Input: part model. Units: mm. Frame: model coordinates. A direction names the side the tool comes from. Round coordinates to 2 decimals unless told otherwise and drop trailing zeros. Order: outer loops, then holes, each group sorted by start corner. A loop starts at its lowest first (then second) coordinate and runs counter-clockwise, first axis right, second up.
Item 1: Cut plane B-B on x = 0. Output: boundary loops of the cut face in (y, z) (3 decimals).
Item 2: First-contact query: pin 1 (6 mm diameter, centred on x = 23.5, y = 11, fed in from +Z); pin 2 (10 mm diameter, centred on y = -2, z = -2, fed in from +X); pin 3 (4 mm diameter, centred on x = -15.5, z = 14, fed in from -Y). Flat tips, straight axial feed; report the tip coordinate or a pass-through.
Item 3: Cut plane A-A on x = 40.5. Output: boundary loops of the cut face in (y, z).
Item 4: Line query: L1, parallel to Y at x = 40, z = -12; L2, parallel to Y at x = 6.5, z = 0; L3, parallel to Y at x = 31, z = 0. Output: solid intervals per line, ascending.
Item 5: Reachability of faces 1 (the conical face through (41.73, 26.92, -0.07)), 2 (the cylindrical face through (42.64, -20.24, 12.9)), 3 (the cylindrical face through (20.012, -11.49, -10.156)) from +Z, -Z, +X, -X, +Y, -Y: full face, straight path, thin tool, end or side. Return the list, or none.
Item 6: Mould query, pull axis Z, two halves, no side actions, for faces 4 (the flat face through (47, -10, -3)), 5 (the cylindrical face through (6.78, 14.36, 34.64)), 6 (the flat face through (-21.5, 24, 8)), 7 (the flat face through (38, -11, 10)). Classes: released by +Z, released by -Z, zero draft, split by the parting line, or undercut.
```python
from build123d import *

# Parameters (mm, degrees)
SKETCH4_R          = 13.125
CUT_EXTRUDE1_DEPTH = 45
FILLET1_R          = 0.4


with BuildPart() as part:
    # Sketch1 → Base-Revolve (revolve)
    with BuildSketch(Plane.XY, mode=Mode.PRIVATE) as base_revolve_sk:
        Polygon((-23, 0), (-23, 37.5), (35.741669751, 37.5), (47, 31), (47, 24), (38, 24), (38, 14), (47, 14), (47, 10), (34, 10), (34, 6), (25, 6), (21.535898385, 0), align=None)
    revolve(base_revolve_sk.sketch.rotate(Axis((-65.592135762, 0, 0), (1, 0, 0)), 90), axis=Axis((-65.592135762, 0, 0), (1, 0, 0)))

    # Sketch2 → Cut-Revolve1 (revolve, cut)
    with BuildSketch(Plane.XY, mode=Mode.PRIVATE) as cut_revolve1_sk:
        Polygon((-23, 36), (-21.5, 36), (-21.5, 31.65), (39, 31.65), (43.416729559, 24), (-23, 24), align=None)
    revolve(cut_revolve1_sk.sketch.rotate(Axis((-29.427152318, 24, 0), (1, 0, 0)), 90), axis=Axis((-29.427152318, 24, 0), (1, 0, 0)), mode=Mode.SUBTRACT)

    # Sketch3 → Cut-Revolve2 (revolve, cut)
    with BuildSketch(Plane.XY, mode=Mode.PRIVATE) as cut_revolve2_sk:
        Polygon((-23, -36), (-21.5, -36), (-21.5, -31.65), (29, -31.65), (33.416729559, -24), (-23, -24), align=None)
    revolve(cut_revolve2_sk.sketch.rotate(Axis((-27.440397351, -24, 0), (1, 0, 0)), 270), axis=Axis((-27.440397351, -24, 0), (1, 0, 0)), mode=Mode.SUBTRACT)

    # Sketch4 → Cut-Extrude1 (cut, symmetric)
    with BuildSketch(Plane.XY):
        Circle(SKETCH4_R)
    extrude(amount=CUT_EXTRUDE1_DEPTH, both=True, mode=Mode.SUBTRACT)

    # Sketch5 → Cut-Revolve3 (revolve, cut)
    with BuildSketch(Plane(origin=(24, 0, 0), x_dir=(0, 0, -1), z_dir=(1, 0, 0)), mode=Mode.PRIVATE) as cut_revolve3_sk:
        Polygon((16.059493946, -34.439695907), (25.122571817, -30.21351329), (24.277335293, -28.400897716), (20.561473366, -30.133632589), (2.811506373, 7.931294466), (-3.975302297, 8.525063287), align=None)
    revolve(cut_revolve3_sk.sketch.rotate(Axis((24, 0, 0), (0, -0.9063077870366493, -0.422618261740701)), 180), axis=Axis((24, 0, 0), (0, -0.9063077870366493, -0.422618261740701)), mode=Mode.SUBTRACT)

    # Fillet1
    fillet1_edges = [part.edges().sort_by_distance(p)[0] for p in [
        (38, -19.458330429, -14.048963553),
    ]]
    fillet(fillet1_edges, radius=FILLET1_R)


solid = part.part
```
From the geometry:
1. outline: (-13.125, -35.128) - (-13.125, 35.128) arc R37.5 ccw to start; (13.125, -35.128) arc R37.5 ccw to (13.125, 35.128) - close; hole circle Ø15.3 at (-24, 0); hole circle Ø15.3 at (24, 0)
2. pin 1: stops at z = 36.64
2. pin 2: stops at x = 34
2. pin 3: stops at y = -35.53
3. outline: circle Ø69.51 at (0, 0); circle Ø28 at (0, 0); hole circle Ø20 at (0, 0); hole (23.47, -5.02) arc R5.05 ccw (long way) to (23.47, 5.02) arc R24 ccw (long way) to start
4. L1: y = -32.92 to -20.78, -7.21 to 7.21, 20.78 to 32.92
4. L2: y = -37.5 to -31.65, -16.35 to -11.4, 11.4 to 16.35, 31.65 to 37.5
4. L3: y = -37.5 to -28.19, -19.81 to -6, 6 to 16.35, 31.65 to 37.5
5. face 1: -X
5. face 2: +X
5. face 3: none
6. face 4: zero draft
6. face 5: split by the parting line
6. face 6: undercut
6. face 7: undercut
